from build123d import *

# Parameters (mm, degrees)
BOSS_EXTRUDE1_DEPTH     = 13
SKETCH3_R               = 14
SKETCH3_R_2             = 6
BOSS_EXTRUDE2_DEPTH     = 17
CUT_EXTRUDE1_DEPTH      = 114.3809949
CUT_EXTRUDE1_DEPTH_BACK = 114.3809949
SKETCH4_R               = 6
FILLET1_R               = 2


with BuildPart() as part:
    # Sketch1 → Revolve1 (revolve)
    with BuildSketch(Plane.XY, mode=Mode.PRIVATE) as revolve1_sk:
        Polygon((0, 0), (22.5, 0), (22.5, -12), (13, -12), (13, -82), (0, -82), align=None)
    revolve(revolve1_sk.sketch.rotate(Axis((0, 0, 0), (0, 1, 0)), 90), axis=Axis((0, 0, 0), (0, 1, 0)))

    # Sketch2 → Boss-Extrude1 (add, symmetric)
    with BuildSketch(Plane(origin=(0, 0, 0), x_dir=(0, 0, -1), z_dir=(1, 0, 0))):
        with BuildLine():
            Line((-18, 5), (18, 5))
            ThreePointArc((18, 5), (22.242640687, 6.757359313), (24, 11))
            Line((24, 11), (24, 29))
            Line((24, 29), (34, 29))
            Line((34, 29), (34, 11))
            ThreePointArc((34, 11), (29.313708499, -0.313708499), (18, -5))
            Line((18, -5), (-18, -5))
            ThreePointArc((-18, -5), (-29.313708499, -0.313708499), (-34, 11))
            Line((-34, 11), (-34, 29))
            Line((-34, 29), (-24, 29))
            Line((-24, 29), (-24, 11))
            ThreePointArc((-24, 11), (-22.242640687, 6.757359313), (-18, 5))
        make_face()
    extrude(amount=BOSS_EXTRUDE1_DEPTH, both=True)

    # Sketch3 → Boss-Extrude2 (add)
    with BuildSketch(Plane.XY.offset(-24)):
        with Locations((0, 29.004149407)):
            Circle(SKETCH3_R)
        with Locations((0, 29.004149407)):
            Circle(SKETCH3_R_2, mode=Mode.SUBTRACT)
    boss_extrude2 = extrude(amount=-BOSS_EXTRUDE2_DEPTH)

    # Mirror1: Boss-Extrude2 across plane
    add(boss_extrude2.mirror(Plane.XY))

    # Sketch4 → Cut-Extrude1 (cut, two sides: drawn at the far end of the back side and taken through both)
    with BuildSketch(Plane(origin=(0, 0, -34), x_dir=(-1, 0, 0), z_dir=(0, 0, -1)).offset(-CUT_EXTRUDE1_DEPTH_BACK)):
        with Locations(Location((0, 29.004149407, 0), (0, 0, 180))):
            Circle(SKETCH4_R)
    extrude(amount=CUT_EXTRUDE1_DEPTH + CUT_EXTRUDE1_DEPTH_BACK, mode=Mode.SUBTRACT)

    # Fillet1
    fillet1_edges = [part.edges().sort_by_distance(p)[0] for p in [
        (0, -12, 13),
    ]]
    fillet(fillet1_edges, radius=FILLET1_R)


solid = part.part
Could you check a few things on this model? Use its own coordinates, in mm. A direction names the side the tool comes from. Coordinates: 2 decimals unless noted, no trailing zeros. Write each loop counter-clockwise with the first axis right and the second up, starting at its lowest first coordinate (ties: lowest second). Pieces come first, ordered by that corner, then holes. Notation, with made-up numbers: (-11.5, 50) - (2.5, 50) arc R30 ccw to (2.5, 88) - close; hole circle Ø11 at (-2, 48.25). An arc over 180 degrees is marked (long way). Put each result on its own line as item: value. Start each with the question number.
Q1. I want a section at B-B on y = 7. Write out the boundary of the cut face in (x, z), plus the area to 3 significant figures.
Q2. I want a section at D-D on z = -27.5. Write out the boundary of the cut face in (x, y), plus the area to 3 significant figures.
Q3. Which directions (+Z, -Z, +X, -X, +Y, -Y) give clear straight access to the entire face, cutting with the end or side of a thin tool? Please do faces 4 (the cylindrical face through (0.182, 6.711, -22.196)), 5 (the cylindrical face through (-1.823, 42.885, 34.27)), 6 (the flat face through (0, 14, 34)).
Q4. I'm going to push flat-ended pins straight in: P1, Ø5, axis at x = 13.5, y = -14, coming from the -Z side; P2, Ø12, axis at y = -18.5, z = 7.5, coming from the -X side; P3, Ø3, axis at x = -17, z = -7, coming from the +Y side; P4, Ø9.5, axis at x = 0, y = 29, coming from the +Z side. Where does each tip first touch, or does it pass through?
Q5. I want a section at C-C on z = 0. Write out the boundary of the cut face in (x, y).
Q6. Please list where these lines run through material, in increasing order: L1, parallel to Y at x = 0, z = -36.5; L2, parallel to Y at x = 17, z = 2.5; L3, parallel to Z at x = 12, y = -74.
Q7. I want a section at A-A on x = 0. Count the separate pieces of the cut face and the enclosed holes in it, plus the area to 3 significant figures.
Q8. Thinking about a two-plate mould opening in Z: for faces 1 (the flat face through (-3.3, 23.7, -24)), 2 (the flat face through (-17, 0, 0)), 3 (the flat face through (0.2, 14.6, -34)), which applies, pulls with the +Z half, pulls with the -Z half, needs draft (parallel to the pull), parting line crosses it, or undercut?
Checks:
1. outline: (-13, -33.49) - (13, -33.49) - (13, -22.47) - (-13, -22.47) - close; (-13, 22.47) - (13, 22.47) - (13, 33.49) - (-13, 33.49) - close
1. area: 573 mm²
2. outline: (-13, -1.87) - (13, -1.87) - (13, 23.81) arc R14 ccw (long way) to (-13, 23.81) - close; hole circle Ø12 at (0, 29)
2. area: 1,000 mm²
3. face 4: +X, -X, +Y
3. face 5: +Z
3. face 6: +Z, -Y
4. P1: z = -19.03
4. P2: x = -12.91
4. P3: y = 0
4. P4: through
5. outline: (-22.5, -12) - (-15, -12) arc R2 cw to (-13, -14) - (-13, -82) - (13, -82) - (13, -14) arc R2 cw to (15, -12) - (22.5, -12) - (22.5, 0) - (13, 0) - (13, 5) - (-13, 5) - (-13, 0) - (-22.5, 0) - close
6. L1: 15 to 23, 35 to 43
6. L2: -12 to 0
6. L3: -5 to 5
7. separate pieces: 3
7. enclosed holes: 0
7. area: 3,470 mm²
8. face 1: undercut
8. face 2: needs draft
8. face 3: pulls with the -Z half
